Read the model definition and answer for the solid it produces. Units are mm, in the model's axes. A direction names the side the tool comes from. Give positions to 0.01 mm unless a question says otherwise; leave off trailing zeros. Order: outer loops, then holes, each group sorted by start corner. A loop starts at its lowest first (then second) coordinate and runs counter-clockwise, first axis right, second up. Notation, with made-up numbers: (-29.5, 47) - (17.5, 47) arc R31 ccw to (17.5, 82) - close; hole circle Ø11 at (30.5, 1). An arc over 180 degrees is marked (long way). Use a Markdown table: item, result. Add a question column.
1. Consider L1, parallel to Z at x = -5, y = 2.6; L2, parallel to X at y = 20, z = -1. Determine where each line is inside the solid, lowest interval first.
2. A cutting plane is placed at C-C on y = 27.4. Determine the outline of the cut face in (x, z).
3. A cutting plane is placed at B-B on x = 5. Determine the outline of the cut face in (y, z).
4. Flat-ended cylindrical pins translate along their axes: P1, Ø1, axis at y = 26, z = 3, coming from the +X side; P2, Ø3, axis at y = 16.5, z = -1.5, coming from the -X side; P3, Ø4, axis at x = -7, z = 0, coming from the +Y side; P4, Ø8, axis at x = 7, y = 5, coming from the -Z side. Find the tip coordinate at first contact, or state that the pin passes through.
5. A cutting plane is placed at A-A on z = 5. Determine the outline of the cut face in (x, y), and give its area (3 significant figures).
6. For a pull along X with two mould halves and no side action, classify faces 1 (the flat face through (0, 2, 9)), 2 (the cylindrical face through (-1, 14, -5)), 3 (the cylindrical face through (7, 2, -5)) as released by +X, released by -X, zero draft, split by the parting line, or undercut.
7. A cutting plane is placed at D-D on x = 0.25. Determine the outline of the cut face in (y, z).
8. Which of the six approach directions +Z, -Z, +X, -X, +Y, -Y give full straight-line access (tool end or side, diameter ignored) to faces 4 (the cylindrical face through (1, 14, -5)), 5 (the cylindrical face through (-1, 10, 5)), 6 (the flat face through (0, 8, -9)), 7 (the flat face through (1.5, 7, 8))?
Autodesk Inventor part; units mm, degrees
ref_plane "YZ Plane" through (0, 0, 0) normal (1, 0, 0) x (0, 1, 0)
ref_plane "XZ Plane" through (0, 0, 0) normal (0, 1, 0) x (-1, 0, 0)
ref_plane "XY Plane" through (0, 0, 0) normal (0, 0, 1) x (1, 0, 0)
sketch "Sketch1" plane through (0, 0, 0) normal (0, 1, 0) x (-1, 0, 0)
  line L0 (-5, 5) -> (5, 5)
  line L1 (5, 5) -> (5, -5)
  line L2 (5, -5) -> (-5, -5)
  line L3 (-5, -5) -> (-5, 5)
  line L4 (-5, 5) -> (5, -5) construction
  line L5 (5, 5) -> (-5, -5) construction
  circle A0 centre (5, 5) radius 2
  circle A1 centre (5, -5) radius 2
  circle A2 centre (-5, 5) radius 2
  circle A3 centre (-5, -5) radius 2
  line L6 (-9, 9) -> (9, 9)
  line L7 (9, 9) -> (9, -9)
  line L8 (9, -9) -> (-9, -9)
  line L9 (-9, -9) -> (-9, 9)
  line L10 (-9, 9) -> (9, -9) construction
  line L11 (9, 9) -> (-9, -9) construction
  point P0 (0, 0)
  dimension "d0" = 10
  dimension "d1" = 10
  dimension "d2" = 4
  dimension "d3" = 4
  dimension "d4" = 4
  dimension "d5" = 4
  dimension "d6" = 18
  dimension "d7" = 18
extrude "Extrusion1" add sketch "Sketch1" along normal blind 4 contours L0 A0 L1 A1 L2 A3 L3 A2 | L6 L7 L8 L9
sketch "Sketch2" plane through (0, 4, 0) normal (0, 1, 0) x (1, 0, 0)
  line L0 (9, 9) -> (-9, 9)
  line L1 (1.5, -9) -> (-1.5, -9)
  line L2 (-1.5, -9) -> (-1.5, 9)
  line L3 (-1.5, 9) -> (1.5, 9)
  line L4 (1.5, 9) -> (1.5, -9)
  line L5 (1.5, -9) -> (-1.5, 9) construction
  line L6 (-1.5, -9) -> (1.5, 9) construction
  circle A0 centre (-5, -5) radius 2
  circle A1 centre (-5, -5) radius 4
  circle A2 centre (-5, 5) radius 2
  circle A3 centre (-5, 5) radius 4
  circle A4 centre (5, -5) radius 2
  circle A5 centre (5, -5) radius 4
  circle A6 centre (5, 5) radius 2
  circle A7 centre (5, 5) radius 4
  point P0 (0, 0)
  point P1 (1.5, -6.9365)
  point P2 (1.5, -3.0635)
  point P3 (1.5, 3.0635)
  point P4 (1.5, 6.9365)
  point P5 (-1.5, 6.9365)
  point P6 (-1.5, 3.0635)
  point P7 (-1.5, -3.0635)
  point P8 (-1.5, -6.9365)
  dimension "d10" = 3
  dimension "d11" = 8
  dimension "d12" = 8
  dimension "d13" = 8
  dimension "d14" = 8
extrude "Extrusion2" add sketch "Sketch2" along normal blind 27 contours L4 A7 A5 L1 L2 A1 A3 L0
sketch "Sketch3" plane through (1.5, 4, 3.0635) normal (1, 0, 0) x (0, 0, -1)
  line L0 (-5.9365, -4) -> (-5.9365, 0)
  line L1 (-5.9365, -4) -> (-5.9365, 23.4)
  line L2 (-5.9365, 0) -> (-5.9365, 27)
  line L3 (-5.9365, 23.4) -> (12.0635, 23.4)
  line L4 (12.0635, 0) -> (12.0635, 27)
  line L5 (12.0635, 23.4) -> (9.5635, 23.4)
  circle A0 centre (9.5635, 23.4) radius 2
  line L6 (5.9635, 19.8) -> (13.1635, 19.8)
  line L7 (13.1635, 19.8) -> (13.1635, 27)
  line L8 (13.1635, 27) -> (5.9635, 27)
  line L9 (5.9635, 27) -> (5.9635, 19.8)
  line L10 (5.9635, 19.8) -> (13.1635, 27) construction
  line L11 (13.1635, 19.8) -> (5.9635, 27) construction
  point P0 (3.0635, -4)
  dimension "d17" = 27.4
  dimension "d18" = 2.5
  dimension "d19" = 4
  dimension "d20" = 7.2
extrude "Extrusion3" add sketch "Sketch3" against normal up to surface (3 mm away) contours A0 L3 L9 L8 L4 | L3 L4 L6 L9 A0 | L4 L8 L7 L6
extrude "Extrusion4" cut sketch "Sketch3" against normal blind 10 contours L3 A0 | L3 A0
chamfer "Chamfer1" distance 10 distance2 25 1 edges at (0, 31, 9) measured on face at (-0.5, 31, -5.7122)
fillet "Fillet1" radius 2 3 edges at (0, 31, -10.1) (0, 23.8, -10.1) (0, 23.8, -9)
properties part number "link1"
Output values:
| question | item | result |
|---|---|---|
| 1 | L1 | -9 to -7, -3 to 3, 7 to 9 |
| 1 | L2 | -1.5 to 1.5 |
| 2 | outline | (-1.5, -10.1) - (1.5, -10.1) - (1.5, -8.5) - (-1.5, -8.5) - close; (-1.5, -4.5) - (1.5, -4.5) - (1.5, 0.44) - (-1.5, 0.44) - close |
| 3 | outline | (0, -9) - (4, -9) - (4, -7) - (0, -7) - close; (0, -3) - (4, -3) - (4, 3) - (0, 3) - close; (0, 7) - (4, 7) - (4, 9) - (0, 9) - close |
| 4 | P1 | through |
| 4 | P2 | x = -1.5 |
| 4 | P3 | y = 4 |
| 4 | P4 | z = -9 |
| 5 | outline | (-9, 0) - (-7, 0) - (-7, 4) - (-9, 4) - close; (-3, 0) - (3, 0) - (3, 4) - (1, 4) - (1, 16) - (-1, 16) - (-1, 4) - (-3, 4) - close; (7, 0) - (9, 0) - (9, 4) - (7, 4) - close |
| 5 | area | 64.0 mm² |
| 6 | face 1 | zero draft |
| 6 | face 2 | released by -X |
| 6 | face 3 | undercut |
| 7 | outline | (0, -9) - (22.01, -9) arc R2 cw to (23.39, -9.55) arc R2 ccw to (24.77, -10.1) - (29, -10.1) arc R2 ccw to (31, -8.1) - (31, -1) - (6, 9) - (0, 9) - close; hole circle Ø4 at (27.4, -6.5) |
| 8 | face 4 | +X |
| 8 | face 5 | -X, +Y |
| 8 | face 6 | -Z, +X, -X, -Y |
| 8 | face 7 | +Z, -Z, +X, +Y |
